```python
from build123d import *

# Parameters (mm, degrees)
SKETCH_1_R          = 26
EXTRUDE_1_DEPTH     = 7
SKETCH_4_R          = 30
SKETCH_4_R_2        = 24
EXTRUDE_4_DEPTH     = 2
SKETCH_5_W          = 24
SKETCH_5_H          = 5
EXTRUDE_5_DEPTH     = 20.7
EXTRUDE_6_DEPTH     = 2
EXTRUDE_7_DEPTH     = 0.56
SKETCH_7_R          = 1.6
CUT_EXTRUDE_1_DEPTH = 16
FILLET_1_R          = 2
FILLET_2_R          = 2
FILLET_3_R          = 2


with BuildPart() as part:
    # 草图1 → 凸台-拉伸1 (new body)
    with BuildSketch(Plane.XY):
        with BuildLine():
            Line((-15.5, -38), (15.5, -38))
            Line((15.5, -38), (15.5, -25.685599078))
            ThreePointArc((15.5, -25.685599078), (0, 30), (-15.5, -25.685599078))
            Line((-15.5, -25.685599078), (-15.5, -38))
        make_face()
        Circle(SKETCH_1_R, mode=Mode.SUBTRACT)
    extrude(amount=EXTRUDE_1_DEPTH)

    # 草图4 → 凸台-拉伸4 (add)
    with BuildSketch(Plane.XY.offset(7)):
        Circle(SKETCH_4_R)
        Circle(SKETCH_4_R_2, mode=Mode.SUBTRACT)
    extrude(amount=EXTRUDE_4_DEPTH)

    # 草图5 → 凸台-拉伸5 (add)
    with BuildSketch(Plane.XY.offset(7)):
        with Locations((0, -35.5)):
            Rectangle(SKETCH_5_W, SKETCH_5_H)
    extrude(amount=EXTRUDE_5_DEPTH)

    # 草图6 → 凸台-拉伸6 (add)
    with BuildSketch(Plane.XY.offset(7)):
        with BuildLine():
            Line((-15.5, -25.685599078), (-15.5, -38))
            Line((-15.5, -38), (-12, -38))
            Line((-12, -38), (-12, -33))
            Line((-12, -33), (12, -33))
            Line((12, -33), (12, -38))
            Line((12, -38), (15.5, -38))
            Line((15.5, -38), (15.5, -25.685599078))
            ThreePointArc((15.5, -25.685599078), (0, -30), (-15.5, -25.685599078))
        make_face()
    extrude(amount=EXTRUDE_6_DEPTH)

    # 草图9 → 凸台-拉伸7 (add)
    with BuildSketch(Plane.XZ.offset(38)):
        Polygon((15.5, 0), (15.5, 9), (12, 9), (12, 27.7), (-12, 27.7), (-12, 9), (-15.5, 9), (-15.5, 0), align=None)
    extrude(amount=EXTRUDE_7_DEPTH)

    # 草图7 → 切除-拉伸1 (cut)
    with BuildSketch(Plane(origin=(0, -33, 0), x_dir=(1, 0, 0), z_dir=(0, 1, 0))):
        with Locations((9, -22.7)):
            Circle(SKETCH_7_R)
        with Locations((-9, -22.7)):
            Circle(SKETCH_7_R)
    extrude(amount=-CUT_EXTRUDE_1_DEPTH, mode=Mode.SUBTRACT)

    # 圆角1
    fillet_1_edges = [part.edges().sort_by_distance(p)[0] for p in [
        (0, -33, 9),
    ]]
    fillet(fillet_1_edges, radius=FILLET_1_R)

    # 圆角2
    fillet_2_edges = [part.edges().sort_by_distance(p)[0] for p in [
        (12, -35.78, 9),
    ]]
    fillet(fillet_2_edges, radius=FILLET_2_R)

    # 圆角3
    fillet_3_edges = [part.edges().sort_by_distance(p)[0] for p in [
        (-12, -35.78, 9),
    ]]
    fillet(fillet_3_edges, radius=FILLET_3_R)


solid = part.part
```
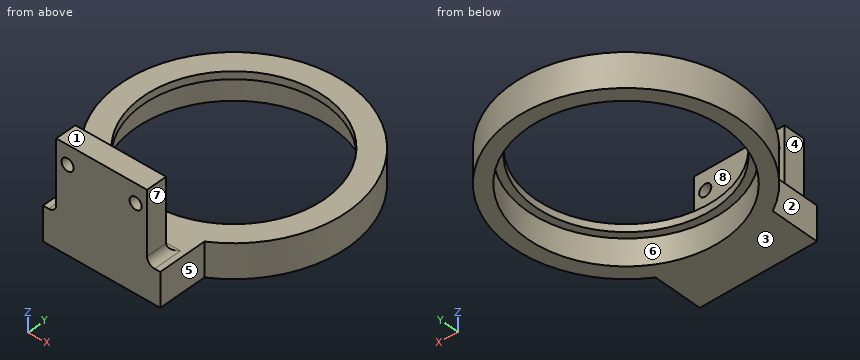
Can you work these out from the model? Positions are in its coordinate system, mm. Face numbers are marked on the shaded views. A direction names the side the tool comes from. Round coordinates to 2 decimals unless told otherwise and drop trailing zeros. Order: outer loops, then holes, each group sorted by start corner. A loop starts at its lowest first (then second) coordinate and runs counter-clockwise, first axis right, second up.
(1) If I drill on L1, parallel to X at y = -34.3, z = 22.7; L2, parallel to Y at x = 0, z = 5.25; L3, parallel to Y at x = 0, z = 8, over which ranges is the centre line in solid material (lowest first)?
Results are:
L1: x = -12 to -10.6, -7.4 to 7.4, 10.6 to 12
L2: y = -38.56 to -26, 26 to 30
L3: y = -38.56 to -24, 24 to 30
(2) On a 3-axis mill with a long thin cutter (end or side, diameter ignored), from which of +Z, -Z, +X, -X, +Y, -Y can I reach the whole of each face in a straight line? I mean the marked faces 1, 2, 3, 4 and 5. Say none if no direction works.
Results are:
face 1: +Z, +X, -X, +Y, -Y
face 2: +Z, -Z, -X, -Y
face 3: -Z, +X, -X, +Y, -Y
face 4: +Z, -X, +Y, -Y
face 5: +Z, -Z, +X, -Y
(3) If we section it at A-A (y = -34): Please give me the cut outline in (x, z), plus the area to 3 significant figures.
Results are:
outline: (-15.5, 0) - (15.5, 0) - (15.5, 9) - (14, 9) arc R2 cw to (12, 11) - (12, 27.7) - (-12, 27.7) - (-12, 11) arc R2 cw to (-14, 9) - (-15.5, 9) - close; hole circle Ø3.2 at (-9, 22.7); hole circle Ø3.2 at (9, 22.7)
area: 713 mm2
(4) If we section it at C-C (y = 0): Please give me the cut outline in (x, z).
Results are:
outline: (-30, 0) - (-26, 0) - (-26, 7) - (-24, 7) - (-24, 9) - (-30, 9) - close; (24, 7) - (26, 7) - (26, 0) - (30, 0) - (30, 9) - (24, 9) - close
(5) If we section it at B-B (x = 20.5): Please give me the cut outline in (y, z).
Results are:
outline: (-21.9, 0) - (-15.99, 0) - (-15.99, 7) - (-12.48, 7) - (-12.48, 9) - (-21.9, 9) - close; (12.48, 7) - (15.99, 7) - (15.99, 0) - (21.9, 0) - (21.9, 9) - (12.48, 9) - close
(6) I'm going to push flat-ended pins straight in: pin 1 (6 mm diameter, centred on y = 8, z = 14.5, fed in from -X); pin 2 (4.5 mm diameter, centred on y = -30.5, z = 3, fed in from +X); pin 3 (1.7 mm diameter, centred on y = -36.5, z = 18.5, fed in from +X); pin 4 (4 mm diameter, centred on x = 9, z = 22.7, fed in from -Y). Where does each tip first touch, or does it pass through?
Results are:
pin 1: passes through
pin 2: stops at x = 15.5
pin 3: stops at x = 12
pin 4: stops at y = -38.56
(7) We'd pull the mould along Y, two halves only. Please class the marked faces 6, 7 and 8: +Y half, -Y half, draft (parallel to the pull), parting line (faces both ways), or undercut.
Results are:
face 6: undercut
face 7: draft
face 8: +Y half
(8) If we section it at D-D (z = 5.5): Please give me the cut outline in (x, y).
Results are:
outline: (-15.5, -38.56) - (15.5, -38.56) - (15.5, -25.69) arc R30 ccw (long way) to (-15.5, -25.69) - close; hole circle Ø52 at (0, 0)
